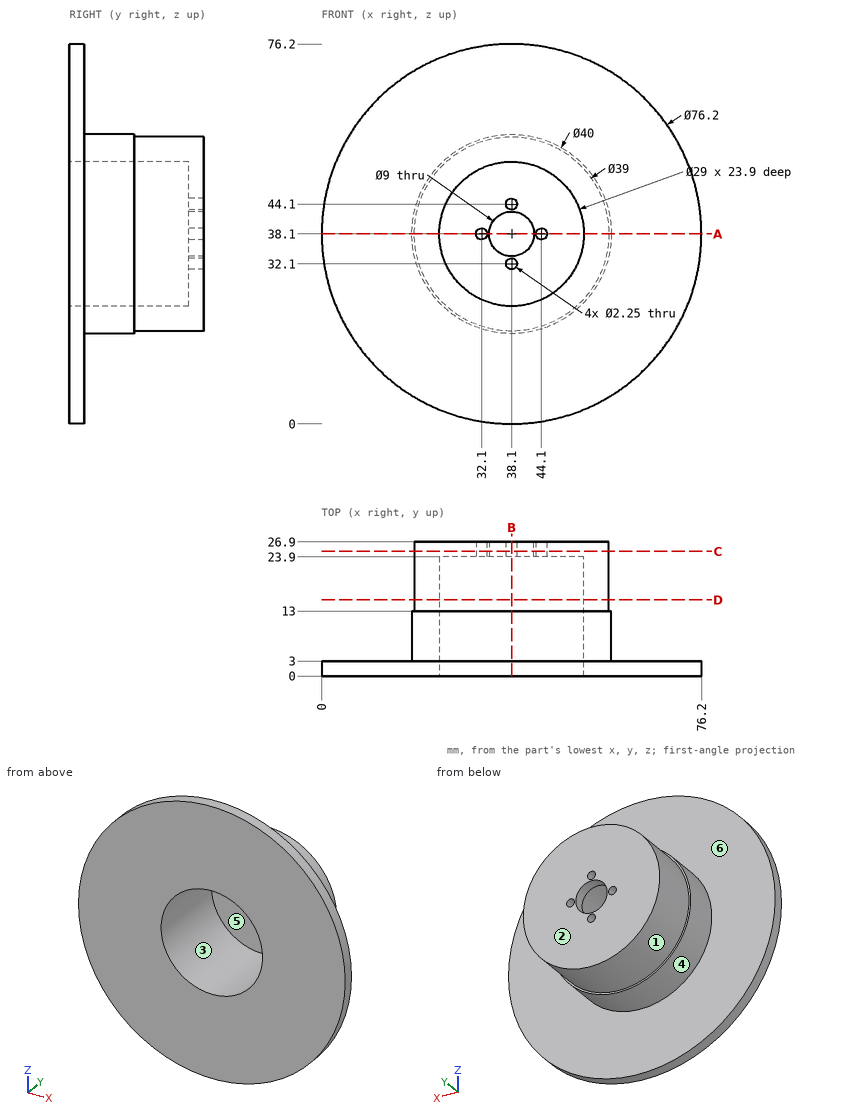
Design review of the part shown in the three views and the two pictorial views. Dimensions are in mm from the part's minimum x, y and z. A direction names the side the tool comes from. Coordinates: 2 decimals unless noted, no trailing zeros. Order: outer loops, then holes, each group sorted by start corner. A loop starts at its lowest first (then second) coordinate and runs counter-clockwise, first axis right, second up. Notation, with made-up numbers: (47, -34) - (84, -34) arc R14 ccw to (84, -23) - close; hole circle Ø11 at (29.5, 41.5). An arc over 180 degrees is marked (long way). Answer as CSV lines item,"result". Start each with the question number.
1) Add section C-C (y = 25). State the section outline as (x, z) points (3 decimals).
2) Add section B-B (x = 38.1). State the section outline as (y, z) points (3 decimals).
3) Add section A-A (z = 38.1). State the section outline as (x, y) points (3 decimals).
4) To check wall thickness, follow line 1 along Z through (x, y) = (38.1, 24.8) (3 decimals); line 2 along X through (y, z) = (18.5, 38.1). State the ranges of each line that lie inside material, in increasing order. Write a range as [from, to].
5) Machinability: for the marked faces 1 and 2, which of the approach directions +Z, -Z, +X, -X, +Y, -Y give a long, thin tool a straight path to every point of the face, cutting with its end or side? Answer none if there is none.
6) Add section D-D (y = 15.25). State the section outline as (x, z) points.
7) Draft analysis for pull direction Z (two halves, no side actions). For the marked faces 3, 4, 5 and 6, state which applies: +Z half, -Z half, draft (parallel to the pull), parting line (faces both ways), or undercut.
8) Insertion check: P1, Ø2.5, axis at x = 32.1, z = 38.1, coming from the -Y side; P2, Ø2, axis at x = 38.1, z = 32.1, coming from the -Y side; P3, Ø1, axis at x = 42.5, y = 5, coming from the +Z side; P4, Ø1.5, axis at y = 12, z = 25, coming from the +X side. Each pin has a flat end and moves straight along its axis. Give the tip position at first contact, or say it passes through.
Result:
1,outline,"circle Ø39 at (38.1, 38.1); hole circle Ø2.25 at (32.1, 38.1); hole circle Ø9 at (38.1, 38.1); hole circle Ø2.25 at (38.1, 32.1); hole circle Ø2.25 at (38.1, 44.1); hole circle Ø2.25 at (44.1, 38.1)"
2,outline,"(0, 0) - (3, 0) - (3, 18.1) - (13, 18.1) - (13, 18.6) - (26.9, 18.6) - (26.9, 30.975) - (23.9, 30.975) - (23.9, 23.6) - (0, 23.6) - close; (0, 52.6) - (23.9, 52.6) - (23.9, 45.225) - (26.9, 45.225) - (26.9, 57.6) - (13, 57.6) - (13, 58.1) - (3, 58.1) - (3, 76.2) - (0, 76.2) - close; (23.9, 33.225) - (26.9, 33.225) - (26.9, 33.6) - (23.9, 33.6) - close; (23.9, 42.6) - (26.9, 42.6) - (26.9, 42.975) - (23.9, 42.975) - close"
3,outline,"(0, 0) - (23.6, 0) - (23.6, 23.9) - (30.975, 23.9) - (30.975, 26.9) - (18.6, 26.9) - (18.6, 13) - (18.1, 13) - (18.1, 3) - (0, 3) - close; (33.225, 23.9) - (33.6, 23.9) - (33.6, 26.9) - (33.225, 26.9) - close; (42.6, 23.9) - (42.975, 23.9) - (42.975, 26.9) - (42.6, 26.9) - close; (45.225, 23.9) - (52.6, 23.9) - (52.6, 0) - (76.2, 0) - (76.2, 3) - (58.1, 3) - (58.1, 13) - (57.6, 13) - (57.6, 26.9) - (45.225, 26.9) - close"
4,line 1,"[18.6, 30.975], [33.225, 33.6], [42.6, 42.975], [45.225, 57.6]"
4,line 2,"[18.6, 23.6], [52.6, 57.6]"
5,face 1,"+Y"
5,face 2,"+Z, -Z, +X, -X, +Y"
6,outline,"circle Ø39 at (38.1, 38.1); hole circle Ø29 at (38.1, 38.1)"
7,face 3,"undercut"
7,face 4,"parting line"
7,face 5,"undercut"
7,face 6,"draft"
8,P1,"y = 23.9"
8,P2,"through"
8,P3,"z = 57.72"
8,P4,"x = 53.83"
